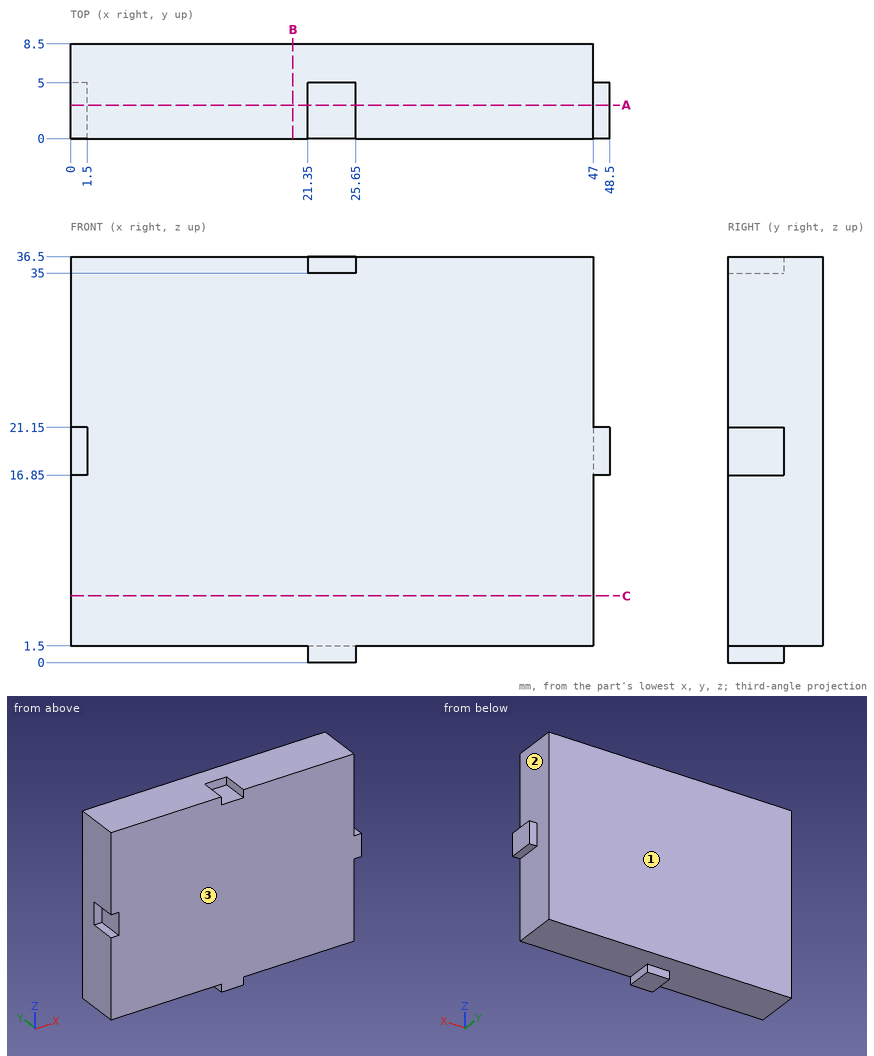
Job drawing, mm, ordinate dimensions from the low corner. One solid piece. Coordinates: 2 decimals unless noted, no trailing zeros. Order: outer loops, then holes, each group sorted by start corner. A loop starts at its lowest first (then second) coordinate and runs counter-clockwise, first axis right, second up. Notation, with made-up numbers: (80, -6.75) - (105, -6.75) arc R8 cw to (105, 7.25) - close; hole circle Ø5 at (57.5, 44.5). An arc over 180 degrees is marked (long way). Return JSON: item names as keys, results as strings. Group by question number.
1) Saw through at C-C, the plane z = 6. Write the cut outline in (x, y), plus the area to 4 significant figures.
2) Saw through at A-A, the plane y = 3. Write the cut outline in (x, z).
3) Mould opens along Y. For the marked faces 1, 2 and 3 say: released by +Y, released by -Y, zero draft, split by the parting line, or undercut.
4) Flat gauge pins, fed straight in: P1, Ø1.6, axis at x = 48, y = 2.5, coming from the +Z side; P2, Ø1.3, axis at x = 23, y = 2.5, coming from the +Z side; P3, Ø1.5, axis at x = 13.5, y = 2.5, coming from the -Z side. Where does each tip first touch, or does it go through?
5) Probe line 1 (Z direction, x = 2, y = 2.5); line 2 (X direction, y = 2.5, z = 11); line 3 (X direction, y = 4.25, z = 17). List the from-to ranges inside material, lowest first. Write a range as from..to.
6) Saw through at B-B, the plane x = 20. Write the cut outline in (y, z).
Values found:
{
 "1": {"outline": "(0, 0) - (47, 0) - (47, 8.5) - (0, 8.5) - close", "area": "399.5 mm²"},
 "2": {"outline": "(0, 1.5) - (21.35, 1.5) - (21.35, 0) - (25.65, 0) - (25.65, 1.5) - (47, 1.5) - (47, 16.85) - (48.5, 16.85) - (48.5, 21.15) - (47, 21.15) - (47, 36.5) - (25.65, 36.5) - (25.65, 35) - (21.35, 35) - (21.35, 36.5) - (0, 36.5) - (0, 21.15) - (1.5, 21.15) - (1.5, 16.85) - (0, 16.85) - close"},
 "3": {"face 1": "released by +Y", "face 2": "zero draft", "face 3": "released by -Y"},
 "4": {"P1": "stops at z = 21.15", "P2": "stops at z = 35", "P3": "stops at z = 1.5"},
 "5": {"line 1": "z = 1.5..36.5", "line 2": "x = 0..47", "line 3": "x = 1.5..48.5"},
 "6": {"outline": "(0, 1.5) - (8.5, 1.5) - (8.5, 36.5) - (0, 36.5) - close"}
}
